Geometry: final body of the model. Coordinates: model frame, mm. A direction names the side the tool comes from. Round coordinates to 2 decimals unless told otherwise and drop trailing zeros. Loops run counter-clockwise (first coordinate to the right, second up) from the corner with the lowest first, then second, coordinate; pieces in that order, holes last. Notation, with made-up numbers: M 27.5,53.5 L 65.5,53.5 A21 ccw 65.5,57.5 Z; hole C 9.25,47 d4. An arc over 180 degrees is marked long. Write each question's results on one line, items separated by ' | '.
```python
from build123d import *

# Parameters (mm, degrees)
F0_W     = 92.1482667327
F0_H     = 127.2523701191
F0_W_2   = 76.1482641101
F0_H_2   = 111.2523674965
F1_DEPTH = 44
F3_W     = 53.4138903022
F3_H     = 15.9167165458
F2_W     = 53.4138903022
F2_H     = 15.9167165458
F4_DEPTH = 146.8
F6_R     = 9.5
F5_R     = 9.5
F7_DEPTH = 171.1


with BuildPart() as f1:
    # F0 (on Top) → F1 (new body)
    with BuildSketch(Plane.XY):
        Rectangle(F0_W, F0_H)
        Rectangle(F0_W_2, F0_H_2, mode=Mode.SUBTRACT)
    extrude(amount=F1_DEPTH)

    # F3 (on face) + F2 (on face) → F4 (cut)
    with BuildSketch(Plane(origin=(-46.0741333663, 0, 0), x_dir=(0, -1, 0), z_dir=(-1, 0, 0))):
        with Locations((0, 36.0416417271)):
            Rectangle(F3_W, F3_H)
    with BuildSketch(Plane.YZ.offset(46.0741333663)):
        with Locations((0, 36.0416417271)):
            Rectangle(F2_W, F2_H)
    extrude(amount=-F4_DEPTH, dir=(-1, 0, 0), mode=Mode.SUBTRACT)

    # F6 (on face) + F5 (on face) → F7 (cut)
    with BuildSketch(Plane(origin=(0, 63.6261850595, 0), x_dir=(-1, 0, 0), z_dir=(0, 1, 0))):
        with Locations((0, 22)):
            Circle(F6_R)
    with BuildSketch(Plane.XZ.offset(63.6261850595)):
        with Locations((0, 22)):
            Circle(F5_R)
    extrude(amount=-F7_DEPTH, dir=(0, 1, 0), mode=Mode.SUBTRACT)


solid = f1.part
```
1. Section A-A (y = -48.5). Output: boundary loops of the cut face in (x, z).
Answer key:
outline: M -46.07,0 L -38.07,0 L -38.07,44 L -46.07,44 Z; M 38.07,0 L 46.07,0 L 46.07,44 L 38.07,44 Z
2. Ray query, probe 1 along Z at (x, y) = (0, -59.5); probe 2 along Y at (x, z) = (-18, 6.5); probe 3 along X at (y, z) = (38.5, 27.5). Return the intervals inside material, ascending.
Answer key:
probe 1: z = 0 to 12.5, 31.5 to 44 | probe 2: y = -63.63 to -55.63, 55.63 to 63.63 | probe 3: x = -46.07 to -38.07, 38.07 to 46.07
3. Section C-C (z = 40). Output: boundary loops of the cut face in (x, y), then the cut area to 3 significant figures.
Answer key:
outline: M -46.07,-63.63 L 46.07,-63.63 L 46.07,-26.71 L 38.07,-26.71 L 38.07,-55.63 L -38.07,-55.63 L -38.07,-26.71 L -46.07,-26.71 Z; M -46.07,26.71 L -38.07,26.71 L -38.07,55.63 L 38.07,55.63 L 38.07,26.71 L 46.07,26.71 L 46.07,63.63 L -46.07,63.63 Z | area: 2,400 mm²
4. Access query for faces 4 (the face through (2.059, -59.57, 12.726)), 5 (the face through (-42, 0, 28.083)), 6 (the face through (-9, 55.626, 17)). Directions: +Z, -Z, +X, -X, +Y, -Y. A direction counts if a zero-diameter tool reaches every point of the face in a straight line with its end or side. Return the directions, or none.
Answer key:
face 4: +Y, -Y | face 5: +Z, +X, -X | face 6: +Z, -Z
5. Pin query (flat end, axial travel): P1, Ø4, axis at x = 43, y = 9, coming from the +Z side; P2, Ø5, axis at y = 23, z = 37, coming from the +X side; P3, Ø22, axis at y = -5.5, z = 28.5, coming from the +X side. Return the tip coordinate at first contact, or that it passes through.
Answer key:
P1: stops at z = 28.08 | P2: passes through | P3: stops at x = 46.07
6. Section B-B (x = -16.5). Output: boundary loops of the cut face in (y, z).
Answer key:
outline: M -63.63,0 L -55.63,0 L -55.63,44 L -63.63,44 Z; M 55.63,0 L 63.63,0 L 63.63,44 L 55.63,44 Z
7. Draft query along Y for faces 1 (the face through (-1, -63.626, 12)), 2 (the face through (2.059, 59.682, 12.726)), 3 (the face through (-42, 26.707, 36)). Return one class per face: pulls with the +Y half, pulls with the -Y half, needs draft (parallel to the pull), parting line crosses it, or undercut.
Answer key:
face 1: pulls with the -Y half | face 2: needs draft | face 3: undercut
8. Section D-D (z = 8.5). Output: boundary loops of the cut face in (x, y).
Answer key:
outline: M -46.07,-63.63 L 46.07,-63.63 L 46.07,63.63 L -46.07,63.63 Z; hole M -38.07,-55.63 L 38.07,-55.63 L 38.07,55.63 L -38.07,55.63 Z
